```python
from build123d import *

# Parameters (mm, degrees)
BOSS_EXTRUDE1_DEPTH     = 35.5
SKETCH2_R               = 12.9
BOSS_EXTRUDE2_DEPTH     = 3
SKETCH3_R               = 4
BOSS_EXTRUDE3_DEPTH     = 26.8
SKETCH4_R               = 12.5
BOSS_EXTRUDE4_DEPTH     = 1
SKETCH5_R               = 8.5
BOSS_EXTRUDE5_DEPTH     = 17.28
CUT_EXTRUDE1_REACH      = 83.306
SKETCH6_R               = 16
CUT_EXTRUDE2_REACH      = 96.36
CUT_EXTRUDE2_END_RADIUS = 16
SKETCH7_R               = 3
CUT_EXTRUDE3_REACH      = 80.627
SKETCH8_R               = 1.25
CUT_EXTRUDE4_REACH      = 79.105
SKETCH9_R               = 1.25
BODY_MOVE_COPY2_ANGLE   = 120


with BuildPart() as part:
    # Sketch1 → Boss-Extrude1 (new body)
    with BuildSketch(Plane.XY):
        Polygon((15.4, 41), (-15.4, 41), (-15.4, 0), (15.4, 0), (15.4, 3), (10.4, 3), (10.4, 38), (15.4, 38), align=None)
    extrude(amount=BOSS_EXTRUDE1_DEPTH)

    # Sketch2 → Boss-Extrude2 (add)
    with BuildSketch(Plane.XY.offset(35.5)):
        with Locations((-2.5, 20.5)):
            Circle(SKETCH2_R)
    extrude(amount=BOSS_EXTRUDE2_DEPTH)

    # Sketch3 → Boss-Extrude3 (add)
    with BuildSketch(Plane.XY.offset(38.5)):
        with Locations((-2.5, 20.5)):
            Circle(SKETCH3_R)
    extrude(amount=BOSS_EXTRUDE3_DEPTH)

    # Sketch4 → Boss-Extrude4 (add)
    with BuildSketch(Plane(origin=(0, 0, 0), x_dir=(-1, 0, 0), z_dir=(0, 0, -1))):
        with Locations((2.5, 20.5)):
            Circle(SKETCH4_R)
    extrude(amount=BOSS_EXTRUDE4_DEPTH)

    # Sketch5 → Boss-Extrude5 (add)
    with BuildSketch(Plane(origin=(0, 0, -1), x_dir=(-1, 0, 0), z_dir=(0, 0, -1))):
        with Locations((2.5, 20.5)):
            Circle(SKETCH5_R)
    extrude(amount=BOSS_EXTRUDE5_DEPTH)

    # Sketch6 → Cut-Extrude1 (cut, up to next)
    with BuildSketch(Plane(origin=(10.4, 0, 0), x_dir=(0, 0, -1), z_dir=(1, 0, 0)), mode=Mode.PRIVATE) as cut_extrude1_sk1:
        with Locations((-17.75, 20.5)):
            Circle(SKETCH6_R)
    cut_extrude1_tool1 = extrude(cut_extrude1_sk1.sketch, amount=-CUT_EXTRUDE1_REACH, mode=Mode.PRIVATE) & part.part
    add(cut_extrude1_tool1.solids().sort_by_distance((10.4, 20.5, 17.75))[0], mode=Mode.SUBTRACT)

    # Cut-Extrude2: up to this cylinder (the profile starts outside it)
    cut_extrude2_end = Plane(origin=(-2.5, 20.5, 17.75), z_dir=(1, 0, 0)) * Cylinder(CUT_EXTRUDE2_END_RADIUS, 225.72, mode=Mode.PRIVATE)
    # Sketch7 → Cut-Extrude2 (cut, up to the surface)
    with BuildSketch(Plane(origin=(0, 0, -18.28), x_dir=(-1, 0, 0), z_dir=(0, 0, -1)), mode=Mode.PRIVATE) as cut_extrude2_sk1:
        with Locations((2.5, 20.5)):
            Circle(SKETCH7_R)
    cut_extrude2_tool1 = extrude(cut_extrude2_sk1.sketch, amount=-CUT_EXTRUDE2_REACH, mode=Mode.PRIVATE) - cut_extrude2_end
    add(cut_extrude2_tool1.solids().sort_by_distance((-2.5, 20.5, -18.28))[0], mode=Mode.SUBTRACT)

    # Sketch8 → Cut-Extrude3 (cut, up to next)
    with BuildSketch(Plane.XZ, mode=Mode.PRIVATE) as cut_extrude3_sk1:
        with Locations(Location((12.9, 30.5, 0), (0, 0, 270))):
            Circle(SKETCH8_R)
    cut_extrude3_tool1 = extrude(cut_extrude3_sk1.sketch, amount=-CUT_EXTRUDE3_REACH, mode=Mode.PRIVATE) & part.part
    # Sketch8 → Cut-Extrude3 (cut, up to next)
    with BuildSketch(Plane.XZ, mode=Mode.PRIVATE) as cut_extrude3_sk2:
        with Locations(Location((12.9, 5.5, 0), (0, 0, 270))):
            Circle(SKETCH8_R)
    cut_extrude3_tool2 = extrude(cut_extrude3_sk2.sketch, amount=-CUT_EXTRUDE3_REACH, mode=Mode.PRIVATE) & part.part
    # Sketch8 → Cut-Extrude3 (cut, up to next)
    with BuildSketch(Plane.XZ, mode=Mode.PRIVATE) as cut_extrude3_sk3:
        with Locations(Location((9.4, 18.45, 0), (0, 0, 270))):
            Circle(SKETCH8_R)
    cut_extrude3_tool3 = extrude(cut_extrude3_sk3.sketch, amount=-CUT_EXTRUDE3_REACH, mode=Mode.PRIVATE) & part.part
    # Sketch8 → Cut-Extrude3 (cut, up to next)
    with BuildSketch(Plane.XZ, mode=Mode.PRIVATE) as cut_extrude3_sk4:
        with Locations(Location((-11.4, 28.65, 0), (0, 0, 270))):
            Circle(SKETCH8_R)
    cut_extrude3_tool4 = extrude(cut_extrude3_sk4.sketch, amount=-CUT_EXTRUDE3_REACH, mode=Mode.PRIVATE) & part.part
    add(cut_extrude3_tool1.solids().sort_by_distance((12.9, 0, 30.5))[0], mode=Mode.SUBTRACT)
    add(cut_extrude3_tool2.solids().sort_by_distance((12.9, 0, 5.5))[0], mode=Mode.SUBTRACT)
    add(cut_extrude3_tool3.solids().sort_by_distance((9.4, 0, 18.45))[0], mode=Mode.SUBTRACT)
    add(cut_extrude3_tool4.solids().sort_by_distance((-11.4, 0, 28.65))[0], mode=Mode.SUBTRACT)

    # Sketch9 → Cut-Extrude4 (cut, up to next)
    with BuildSketch(Plane.XZ.offset(-38), mode=Mode.PRIVATE) as cut_extrude4_sk1:
        with Locations(Location((12.9, 30.5, 0), (0, 0, 270))):
            Circle(SKETCH9_R)
    cut_extrude4_tool1 = extrude(cut_extrude4_sk1.sketch, amount=-CUT_EXTRUDE4_REACH, mode=Mode.PRIVATE) & part.part
    # Sketch9 → Cut-Extrude4 (cut, up to next)
    with BuildSketch(Plane.XZ.offset(-38), mode=Mode.PRIVATE) as cut_extrude4_sk2:
        with Locations(Location((12.9, 5.5, 0), (0, 0, 270))):
            Circle(SKETCH9_R)
    cut_extrude4_tool2 = extrude(cut_extrude4_sk2.sketch, amount=-CUT_EXTRUDE4_REACH, mode=Mode.PRIVATE) & part.part
    add(cut_extrude4_tool1.solids().sort_by_distance((12.9, 38, 30.5))[0], mode=Mode.SUBTRACT)
    add(cut_extrude4_tool2.solids().sort_by_distance((12.9, 38, 5.5))[0], mode=Mode.SUBTRACT)


with BuildPart() as part_1:
    # Body-Move/Copy1: moved
    add(part.part.moved(Location((2.5, -20.5, -17.75))))


with BuildPart() as part_2:
    # Body-Move/Copy2: moved
    add(part_1.part.rotate(Axis((0, 0, 0), (0.5773502691896272, 0.5773502691896252, -0.5773502691896252)), BODY_MOVE_COPY2_ANGLE))


solid = part_2.part
```
CAD build for the part. Positions are in the model's coordinates, mm. A direction names the side the tool comes from. Give positions to 0.01 mm unless a question says otherwise; leave off trailing zeros. Loops run counter-clockwise (first coordinate to the right, second up) from the corner with the lowest first, then second, coordinate; pieces in that order, holes last. Notation, with made-up numbers: (13.5, -4) -> (56.5, -4) arc R20 cw to (56.5, 6) -> close; hole circle Ø8 at (-35.5, 66). An arc over 180 degrees is marked (long way). Use a Markdown table: item, result.
1. Slice it at B-B (x = 14). List the corners of the cut face in (y, z), plus the area to 3 significant figures.
Check result:
| item | result |
|---|---|
| outline | (-17.75, -12.9) -> (-7.75, -12.9) -> (-7.75, 12.9) -> (-17.75, 12.9) -> close; (7.75, -12.9) -> (17.75, -12.9) -> (17.75, 12.9) -> (7.75, 12.9) -> close |
| area | 516 mm^2 |
2. Slice it at D-D (z = 0). List the corners of the cut face in (x, y), plus the area to 3 significant figures.
Check result:
| item | result |
|---|---|
| outline | (-20.5, -17.75) -> (-12.9, -17.75) -> (-12.9, -20.75) -> (-4, -20.75) -> (-4, -47.55) -> (4, -47.55) -> (4, -20.75) -> (12.9, -20.75) -> (12.9, -17.75) -> (20.5, -17.75) -> (20.5, 17.75) -> (12.5, 17.75) -> (12.5, 18.75) -> (8.5, 18.75) -> (8.5, 36.03) -> (3, 36.03) -> (3, 15.72) arc R16 cw (long way) to (-3, 15.72) -> (-3, 36.03) -> (-8.5, 36.03) -> (-8.5, 18.75) -> (-12.5, 18.75) -> (-12.5, 17.75) -> (-20.5, 17.75) -> close |
| area | 1,140 mm^2 |
3. Slice it at C-C (y = 12.25). List the corners of the cut face in (x, z).
Check result:
| item | result |
|---|---|
| outline | (-20.5, -17.9) -> (-17.5, -17.9) -> (-17.5, -16.65) -> (-20.5, -16.65) -> close; (-20.5, -14.15) -> (-17.5, -14.15) -> (-17.5, -12.9) -> (-10.29, -12.9) -> (-10.29, 12.9) -> (-20.5, 12.9) -> close; (10.29, -12.9) -> (17.5, -12.9) -> (17.5, -14.15) -> (20.5, -14.15) -> (20.5, 12.9) -> (10.29, 12.9) -> close; (17.5, -17.9) -> (20.5, -17.9) -> (20.5, -16.65) -> (17.5, -16.65) -> close |
4. Mould opens along Y. For faces 6 (the cylindrical face through (18.98, -12.91, -16.64)), 7 (the flat face through (0, -47.55, 0)), 8 (the cylindrical face through (-19.02, 12.09, -16.64)), 9 (the cylindrical face through (-11.445, -19.229, -5.953)) say: pulls with the +Y half, pulls with the -Y half, needs draft (parallel to the pull), parting line crosses it, or undercut.
Check result:
| item | result |
|---|---|
| face 6 | undercut |
| face 7 | pulls with the -Y half |
| face 8 | undercut |
| face 9 | needs draft |
5. Flat gauge pins, fed straight in: pin 1 (5 mm diameter, centred on x = 3.5, y = -15.5, fed in from -Z); pin 2 (2 mm diameter, centred on x = -1, y = -24.5, fed in from -Z); pin 3 (6 mm diameter, centred on x = 10.5, z = 1, fed in from -Y). Where does each tip first touch, or does it go through?
Check result:
| item | result |
|---|---|
| pin 1 | stops at z = -12.9 |
| pin 2 | stops at z = -4 |
| pin 3 | stops at y = -20.75 |
6. Which spindle directions (+Z, -Z, +X, -X, +Y, -Y) get a long thin tool onto all of the face, cutting with end or side? Do faces 1 (the flat face through (-15, -17.75, -2)), 2 (the flat face through (17.5, 0, -15)), 3 (the flat face through (15, -17.75, -2)), 4 (the cylindrical face through (-3.905, -33.962, 0.867)), 5 (the cylindrical face through (-16.65, -12.15, 8.85)). Say none if no direction does.
Check result:
| item | result |
|---|---|
| face 1 | -X, -Y |
| face 2 | -Z, +Y, -Y |
| face 3 | +X, -Y |
| face 4 | -Y |
| face 5 | -X |
7. Wall check: L1, parallel to Z at x = 18.5, y = 12.25; L2, parallel to X at y = 0, z = -1.5; L3, parallel to Y at x = -16.5, z = 8.9. Give the ranges that are in metal, low to high. Write a range as [from, to].
Check result:
| item | result |
|---|---|
| L1 | z = [-17.9, -16.65], [-14.15, 12.9] |
| L2 | x = [-20.5, -16], [16, 20.5] |
| L3 | y = [-17.75, -12.15], [-9.65, 17.75] |
8. Slice it at A-A (z = -15.4). List the corners of the cut face in (x, y).
Check result:
| item | result |
|---|---|
| outline | (-20.5, -17.75) -> (-17.5, -17.75) -> (-17.5, -14) -> (-20.5, -14) -> close; (-20.5, -11.5) -> (-17.5, -11.5) -> (-17.5, 11) -> (-20.5, 11) -> close; (-20.5, 13.5) -> (-17.5, 13.5) -> (-17.5, 17.75) -> (-20.5, 17.75) -> close; (17.5, -17.75) -> (20.5, -17.75) -> (20.5, -14) -> (17.5, -14) -> close; (17.5, -11.5) -> (20.5, -11.5) -> (20.5, 11) -> (17.5, 11) -> close; (17.5, 13.5) -> (20.5, 13.5) -> (20.5, 17.75) -> (17.5, 17.75) -> close |
